Part model, mm, in its own coordinate system. A direction names the side the tool comes from. Coordinates: 2 decimals unless noted, no trailing zeros. Loops run counter-clockwise (first coordinate to the right, second up) from the corner with the lowest first, then second, coordinate; pieces in that order, holes last. Notation, with made-up numbers: M 66.5,-24 L 73.5,-24 A32 ccw 73.5,15 Z; hole C -31.5,31.5 d10. An arc over 180 degrees is marked long. Use a Markdown table: item, result. Add a question column.
1) Band-saw the part on D-D (y = 22.5). List the corners of the cut face in (x, z), plus the area to 4 significant figures.
2) Tool access for faces 1 (the flat face through (0.52, 23.55, 73.07)), 2 (the flat face through (58.554, -12, 41)): list every direction of +Z, -Z, +X, -X, +Y, -Y with a clear straight run to the whole face (end or side of a thin tool).
3) Band-saw the part on A-A (z = 14). List the corners of the cut face in (x, y).
4) Wall check: probe 1 along X at (y, z) = (12, 62); probe 2 along Y at (x, z) = (57.5, 53.5); probe 3 along Y at (x, z) = (-5.5, 71). Give the ranges that are in metal, low to high. Write a range as from..to.
5) Pin check, flat tip, straight feed: pin 1 Ø1.5 at (x, y) = (7, 3) entering from +Z. Stop position of the tip, or through.
from build123d import *

# Parameters (mm, degrees)
F0_W     = 127
F0_H     = 76.2
F1_DEPTH = 76.2
F2_T     = -6.35
F3_SIZE  = 6.34999


# Not quite as in the source:
# - a fillet or chamfer is up to 0.001 mm smaller than in the source, because OpenCascade refuses the exact size


with BuildPart() as f1:
    # F0 (on Top) → F1 (new body)
    with BuildSketch(Plane.XY):
        with Locations((1.4040806768, -11.3298352808)):
            Rectangle(F0_W, F0_H)
    extrude(amount=F1_DEPTH)

    # F2
    f2_openings = [f1.faces().sort_by_distance(p)[0] for p in [
        (1.404081, -11.329835, 76.2),
    ]]
    offset(amount=F2_T, openings=f2_openings)

    # F3 (size 6.35 in the source; OpenCascade refuses exactly that, so slightly less here)
    f3_edges = [f1.edges().sort_by_distance(p)[0] for p in [
        (1.404081, -49.429835, 76.2),
        (1.404081, 26.770165, 76.2),
        (64.904081, -11.329835, 76.2),
        (-62.095919, -11.329835, 76.2),
    ]]
    chamfer(f3_edges, length=F3_SIZE)


solid = f1.part
Entries:
| question | item | result |
|---|---|---|
| 1 | outline | M -62.1,0 L 64.9,0 L 64.9,69.85 L 60.63,74.12 L -57.83,74.12 L -62.1,69.85 Z |
| 1 | area | 9,395 mm2 |
| 2 | face 1 | +Z, +X, -X, +Y |
| 2 | face 2 | +Z |
| 3 | outline | M -62.1,-49.43 L 64.9,-49.43 L 64.9,26.77 L -62.1,26.77 Z; hole M -55.75,-43.08 L 58.55,-43.08 L 58.55,20.42 L -55.75,20.42 Z |
| 4 | probe 1 | -62.1..-55.75, 58.55..64.9 |
| 4 | probe 2 | -49.43..-43.08, 20.42..26.77 |
| 4 | probe 3 | -48.28..-43.08, 20.42..25.62 |
| 5 | pin 1 | z = 6.35 |
